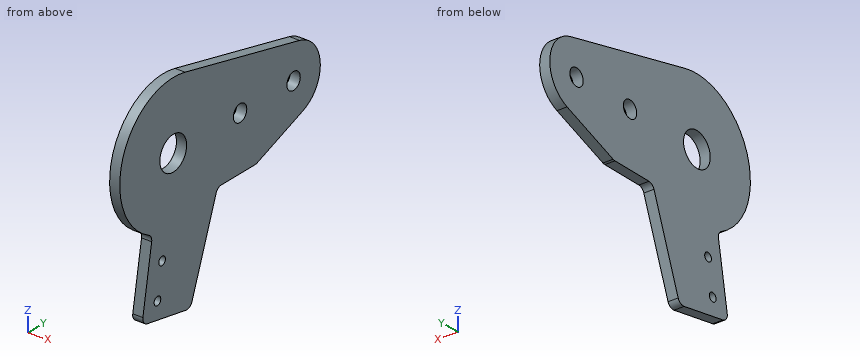
```python
from build123d import *

# Parameters (mm, degrees)
SKETCH1_R           = 5
SKETCH1_R_2         = 2.5
SKETCH1_R_3         = 1.25
BOSS_EXTRUDE1_DEPTH = 3
FILLET1_R           = 2


with BuildPart() as part:
    # Sketch1 → Boss-Extrude1 (new body)
    with BuildSketch(Plane(origin=(0, 0, 0), x_dir=(0, 0, -1), z_dir=(1, 0, 0))):
        with BuildLine():
            Line((-59.74996043, 17.222222222), (-69.499920861, -25.555555556))
            ThreePointArc((-69.499920861, -25.555555556), (-56.144118615, -49.032861226), (-31.582037919, -37.796067776))
            Line((-31.582037919, -37.796067776), (-9.457329759, -41.697250765))
            Line((-9.457329759, -41.697250765), (-6.26133088, -23.571840424))
            Line((-6.26133088, -23.571840424), (-34, -13.475790526))
            Line((-34, -13.475790526), (-34, 1))
            Line((-34, 1), (-40.649042421, 18.543951518))
            ThreePointArc((-40.649042421, 18.543951518), (-50.690320869, 24.9761444), (-59.74996043, 17.222222222))
        make_face()
        with Locations((-50, -30)):
            Circle(SKETCH1_R, mode=Mode.SUBTRACT)
        with Locations((-50, 15)):
            Circle(SKETCH1_R_2, mode=Mode.SUBTRACT)
        with Locations((-50, -5)):
            Circle(SKETCH1_R_2, mode=Mode.SUBTRACT)
        with Locations((-23.361205166, -34.168489335)):
            Circle(SKETCH1_R_3, mode=Mode.SUBTRACT)
        with Locations((-13.513127636, -35.904971111)):
            Circle(SKETCH1_R_3, mode=Mode.SUBTRACT)
    extrude(amount=BOSS_EXTRUDE1_DEPTH)

    # Fillet1
    fillet1_edges = [part.edges().sort_by_distance(p)[0] for p in [
        (1.5, 1, 34),
        (1.5, -13.475790526, 34),
        (1.5, -23.571840424, 6.26133088),
        (1.5, -41.697250765, 9.457329759),
        (1.5, -37.796067776, 31.582037919),
    ]]
    fillet(fillet1_edges, radius=FILLET1_R)


solid = part.part
```
Here's how the part is built. I have some questions about the finished solid (model axes, mm). Round coordinates to 2 decimals unless told otherwise and drop trailing zeros. Write each loop counter-clockwise with the first axis right and the second up, starting at its lowest first coordinate (ties: lowest second). Pieces come first, ordered by that corner, then holes.
Q1. If we section it at B-B on y = 15: Write out the boundary of the cut face in (x, z).
Q2. If we section it at C-C on y = -5: Write out the boundary of the cut face in (x, z), plus the area to 3 significant figures.
Q3. If we section it at A-A on x = 2: Write out the boundary of the cut face in (y, z).
Q4. If we section it at D-D on z = 63: Write out the boundary of the cut face in (x, y), plus the area to 3 significant figures.
Q5. Will these pins go through, and if not, where does the flat tip stop? P1, Ø1.5, axis at x = 0.5, y = -36.5, coming from the -Z side; P2, Ø0.9, axis at x = 1.5, y = -3.5, coming from the -Z side; P3, Ø2, axis at y = -34.17, z = 23.36, coming from the -X side.
Q6. Please list where these lines run through material, in increasing order: probe 1 along Y at (x, z) = (0.8, 50); probe 2 along Z at (x, y) = (1.6, 14); probe 3 along Z at (x, y) = (0.4, 13.5).
Answer below:
1. outline: (0, 39.31) - (3, 39.31) - (3, 47.5) - (0, 47.5) - close; (0, 52.5) - (3, 52.5) - (3, 60.26) - (0, 60.26) - close
2. outline: (0, 34) - (3, 34) - (3, 47.5) - (0, 47.5) - close; (0, 52.5) - (3, 52.5) - (3, 64.81) - (0, 64.81) - close
2. area: 77.4 mm2
3. outline: (-41.35, 11.43) arc R2 ccw to (-39.73, 9.11) - (-25.22, 6.55) arc R2 ccw to (-23, 7.84) - (-13.95, 32.68) arc R2 cw to (-12.08, 34) - (0.63, 34) arc R2 ccw to (1.34, 34.13) - (18.54, 40.65) arc R10 ccw to (17.22, 59.75) - (-25.56, 69.5) arc R20 ccw to (-39.12, 32.2) arc R2 cw to (-38.06, 30.07) - close; hole circle Ø2.5 at (-35.9, 13.51); hole circle Ø2.5 at (-34.17, 23.36); hole circle Ø10 at (-30, 50); hole circle Ø5 at (-5, 50); hole circle Ø5 at (15, 50)
4. outline: (0, -45.2) - (3, -45.2) - (3, 2.96) - (0, 2.96) - close
4. area: 144 mm2
5. P1: stops at z = 8.41
5. P2: stops at z = 34
5. P3: passes through
6. probe 1: y = -50 to -35, -25 to -7.5, -2.5 to 12.5, 17.5 to 25
6. probe 2: z = 38.93 to 47.71, 52.29 to 60.48
6. probe 3: z = 38.74 to 48, 52 to 60.6
